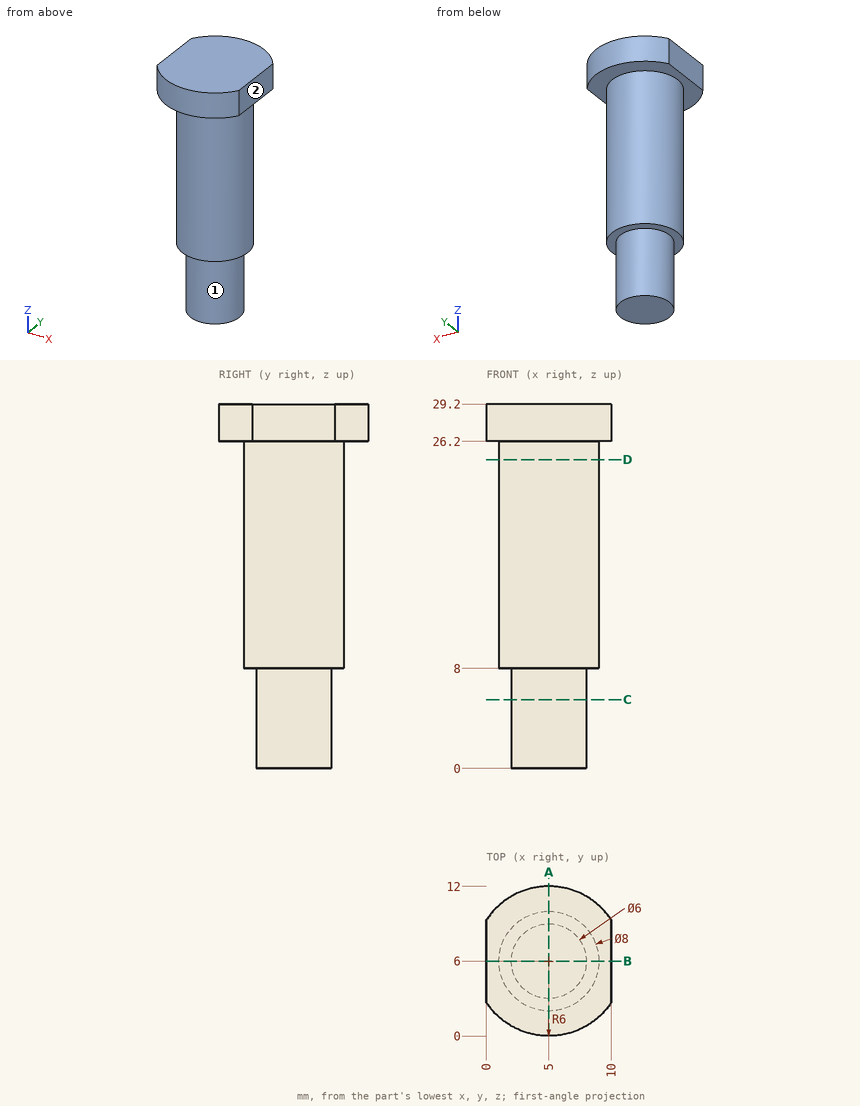
Here's the drawing with two shaded views (mm, measured from the low corner). I have some questions. A direction names the side the tool comes from. Give positions to 0.01 mm unless a question says otherwise; leave off trailing zeros. Loops run counter-clockwise (first coordinate to the right, second up) from the corner with the lowest first, then second, coordinate; pieces in that order, holes last. Notation, with made-up numbers: (55.25, 74.5) -> (64.25, 74.5) arc R22 cw to (64.25, 87.5) -> close; hole circle Ø11 at (-22.75, -4.75). An arc over 180 degrees is marked (long way). Use one line per item in the form item = value.
1) I need wall thicknesses on line 1 along Z through (x, y) = (0.5, 8.5); line 2 along Z through (x, y) = (7.5, 4.25); line 3 along Y through (x, z) = (6.5, 11.5). Which ranges of each line are inside material? Lowest first, please.
Answers:
line_1 = 26.2 to 29.2
line_2 = 8 to 29.2
line_3 = 2.29 to 9.71
2) If we section it at C-C (z = 5.5): Please give me the cut outline in (x, y).
Answers:
outline = circle Ø6 at (5, 6)
3) Will these pins go through, and if not, where does the flat tip stop? pin 1 (1 mm diameter, centred on x = 6, z = 21, fed in from -Y); pin 2 (1 mm diameter, centred on y = 5.5, z = 15, fed in from +X); pin 3 (5 mm diameter, centred on x = 7, z = 6.5, fed in from +Y).
Answers:
pin_1 = 2.03
pin_2 = 9
pin_3 = 10
4) If we section it at D-D (z = 24.75): Please give me the cut outline in (x, y), plus the area to 3 significant figures.
Answers:
outline = circle Ø8 at (5, 6)
area = 50.3 mm²
5) If we section it at A-A (x = 5): Please give me the cut outline in (y, z).
Answers:
outline = (0, 26.2) -> (2, 26.2) -> (2, 8) -> (3, 8) -> (3, 0) -> (9, 0) -> (9, 8) -> (10, 8) -> (10, 26.2) -> (12, 26.2) -> (12, 29.2) -> (0, 29.2) -> close
6) If we section it at B-B (y = 6): Please give me the cut outline in (x, z), plus the area to 3 significant figures.
Answers:
outline = (0, 26.2) -> (1, 26.2) -> (1, 8) -> (2, 8) -> (2, 0) -> (8, 0) -> (8, 8) -> (9, 8) -> (9, 26.2) -> (10, 26.2) -> (10, 29.2) -> (0, 29.2) -> close
area = 224 mm²
7) For the marked faces 1 and 2, which set-ups out of +Z, -Z, +X, -X, +Y, -Y let a thin tool reach every point of the face, with its end or its side?
Answers:
face_1 = -Z
face_2 = +Z, -Z, +X, +Y, -Y
